CAD build for the part. Positions are in the model's coordinates, mm. Round coordinates to 2 decimals unless told otherwise and drop trailing zeros. Loops run counter-clockwise (first coordinate to the right, second up) from the corner with the lowest first, then second, coordinate; pieces in that order, holes last. Notation, with made-up numbers: M -12.75,16 L 27.25,16 A20 ccw 27.25,30 Z; hole C 75,7.25 d9. An arc over 180 degrees is marked long. One line per item, written item: value. Start each with the question number.
from build123d import *

# Parameters (mm, degrees)
F0_R          = 46.355
F1_DEPTH      = 25.4
F2_START      = 1.778
F2_DEPTH      = 21.844
F3_DEPTH      = 23.622
F3_DEPTH_BACK = 1.778


with BuildPart() as f1:
    # F0 (on Top) → F1 (new body)
    with BuildSketch(Plane.XY):
        Circle(F0_R)
        with BuildLine():
            ThreePointArc((-44.45, 0), (0, 44.45), (44.45, 0))
            ThreePointArc((44.45, 0), (1.016, -44.4383870544), (-44.4035542857, -2.0314691225))
            ThreePointArc((-44.4035542857, -2.0314691225), (-44.4383870544, -1.016), (-44.45, 0))
        make_face(mode=Mode.SUBTRACT)
    extrude(amount=F1_DEPTH)

    # F0 (on Top) → F2 (join)
    with BuildSketch(Plane.XY.offset(F2_START)):
        with BuildLine():
            ThreePointArc((-44.4035542857, -2.0314691225), (-43.4110425816, -0.9925117041), (-44.45, 0))
            ThreePointArc((-44.45, 0), (-44.4383870544, -1.016), (-44.4035542857, -2.0314691225))
        make_face()
    extrude(amount=F2_DEPTH)

    # F3 (add, two sides): a face of the model
    f3_faces = [f1.faces().sort_by_distance(p)[0] for p in [
        (-43.9998730556, -1.0059742036, 23.622),
    ]]
    extrude(f3_faces, amount=F3_DEPTH)
    extrude(f3_faces, amount=-F3_DEPTH_BACK)


solid = f1.part
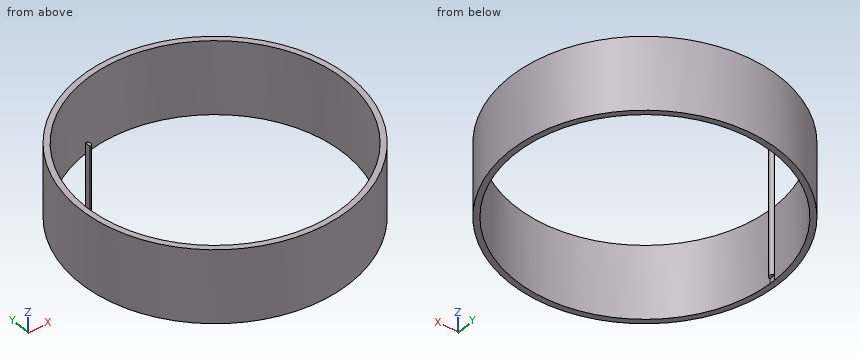
(1) Probe L1, parallel to Y at x = 0, z = 9.5 (3 decimals); L2, parallel to Y at x = 6, z = 16.5; L3, parallel to X at y = -24.5, z = 4. List the from-to ranges inside material, lowest first.
(2) Slice it at C-C, the plane z = 7.5. List the corners of the cut face in (x, y) (3 decimals), and give its area (3 significant figures).
(3) Slice it at A-A, the plane x = 0. List the corners of the cut face in (y, z) (3 decimals), and give its area (3 significant figures).
(4) Slice it at B-B, the plane y = -10.5. List the corners of the cut face in (x, z).
(5) Flat gauge pins, fed straight in: P1, Ø8, axis at y = 4, z = 18, coming from the -X side (3 decimals); P2, Ø10, axis at y = 7, z = 5, coming from the -X side; P3, Ø5, axis at x = -4, z = 17, coming from the +Y side; P4, Ø2, axis at x = 10.5, z = 24.5, coming from the -Y side. Where does each tip first touch, or does it go through?
Check result:
1. L1: y = -46.355 to -44.45, 44.45 to 46.355
1. L2: y = -45.97 to -44.04, 44.04 to 45.97
1. L3: x = -39.35 to -37.09, 37.09 to 39.35
2. outline: C 0,0 d92.71; hole M -44.45,0 A1.016 cw -44.404,-2.031 A44.45 ccw long Z
2. area: 545 mm^2
3. outline: M -46.355,0 L -44.45,0 L -44.45,25.4 L -46.355,25.4 Z; M 44.45,0 L 46.355,0 L 46.355,25.4 L 44.45,25.4 Z
3. area: 96.8 mm^2
4. outline: M -45.15,0 L -43.19,0 L -43.19,25.4 L -45.15,25.4 Z; M 43.19,0 L 45.15,0 L 45.15,25.4 L 43.19,25.4 Z
5. P1: stops at x = -46.355
5. P2: stops at x = -46.31
5. P3: stops at y = 46.33
5. P4: stops at y = -45.37
